```python
from build123d import *

# Parameters (mm, degrees)
SKETCH1_W                                       = 60
SKETCH1_H                                       = 120
BOSS_EXTRUDE1_DEPTH                             = 6.54
BOSS_EXTRUDE4_DEPTH                             = 27
SKETCH10_W                                      = 6.54
SKETCH10_H                                      = 45
BOSS_EXTRUDE5_DEPTH                             = 20
SKETCH17_W                                      = 60
SKETCH17_H                                      = 40
BOSS_EXTRUDE6_DEPTH                             = 29
CUT_EXTRUDE1_REACH                              = 72
SKETCH18_RX                                     = 20.2
SKETCH18_RY                                     = 12
CUT_EXTRUDE2_REACH                              = 57.54
SKETCH21_W                                      = 40.3853088
SKETCH21_H                                      = 40
SKETCH23_W                                      = 2
SKETCH23_H                                      = 36
CUT_EXTRUDE3_DEPTH                              = 9
SKETCH24_W                                      = 2
SKETCH24_H                                      = 36
CUT_EXTRUDE4_DEPTH                              = 9
CSK_FOR_M3_FLAT_HEAD_MACHINE_SCREW4_D           = 4.93
CSK_FOR_M3_FLAT_HEAD_MACHINE_SCREW4_DEPTH       = 6.54
CSK_FOR_M3_FLAT_HEAD_MACHINE_SCREW4_CSINK_D     = 12
CSK_FOR_M3_FLAT_HEAD_MACHINE_SCREW4_CSINK_ANGLE = 90
CSK_FOR_M3_FLAT_HEAD_MACHINE_SCREW5_D           = 4.93
CSK_FOR_M3_FLAT_HEAD_MACHINE_SCREW5_DEPTH       = 6.54
CSK_FOR_M3_FLAT_HEAD_MACHINE_SCREW5_CSINK_D     = 12
CSK_FOR_M3_FLAT_HEAD_MACHINE_SCREW5_CSINK_ANGLE = 90


with BuildPart() as part:
    # Sketch1 → Boss-Extrude1 (new body)
    with BuildSketch(Plane.XY):
        Rectangle(SKETCH1_W, SKETCH1_H)
    extrude(amount=BOSS_EXTRUDE1_DEPTH)

    # Sketch7 → Boss-Extrude4 (add)
    with BuildSketch(Plane.XY.offset(6.54)):
        with BuildLine():
            Line((-30, 44.483314774), (-30, 29.516685226))
            ThreePointArc((-30, 29.516685226), (-16, 37), (-30, 44.483314774))
        make_face()
    extrude(amount=BOSS_EXTRUDE4_DEPTH)

    # Sketch10 → Boss-Extrude5 (add)
    with BuildSketch(Plane(origin=(0, 0, 0), x_dir=(-1, 0, 0), z_dir=(0, 0, -1))):
        with Locations((23.27, -2.5)):
            Rectangle(SKETCH10_W, SKETCH10_H)
        with Locations((-23.27, -2.5)):
            Rectangle(SKETCH10_W, SKETCH10_H)
    extrude(amount=BOSS_EXTRUDE5_DEPTH)

    # Sketch17 → Boss-Extrude6 (add)
    with BuildSketch(Plane.XY.offset(6.54)):
        with Locations((0, -10)):
            Rectangle(SKETCH17_W, SKETCH17_H)
    extrude(amount=BOSS_EXTRUDE6_DEPTH)

    # Sketch18 → Cut-Extrude1 (cut, up to next)
    with BuildSketch(Plane(origin=(0, 10, 0), x_dir=(1, 0, 0), z_dir=(0, 1, 0)), mode=Mode.PRIVATE) as cut_extrude1_sk1:
        with Locations(Location((4.192654401, -20.096314851), (0, 0, 1.545214336))):
            Ellipse(SKETCH18_RX, SKETCH18_RY)
    cut_extrude1_tool1 = extrude(cut_extrude1_sk1.sketch, amount=-CUT_EXTRUDE1_REACH, mode=Mode.PRIVATE) & part.part
    add(cut_extrude1_tool1.solids().sort_by_distance((4.192654, 10, 20.096315))[0], mode=Mode.SUBTRACT)

    # Sketch21 → Cut-Extrude2 (cut, up to next)
    with BuildSketch(Plane.XY.offset(35.54), mode=Mode.PRIVATE) as cut_extrude2_sk1:
        with Locations((4.1926544, -10)):
            Rectangle(SKETCH21_W, SKETCH21_H)
    cut_extrude2_tool1 = extrude(cut_extrude2_sk1.sketch, amount=-CUT_EXTRUDE2_REACH, mode=Mode.PRIVATE) & part.part
    add(cut_extrude2_tool1.solids().sort_by_distance((4.192654, -10, 35.54))[0], mode=Mode.SUBTRACT)

    # Sketch23 → Cut-Extrude3 (cut)
    with BuildSketch(Plane(origin=(-16, 0, 0), x_dir=(0, 0, -1), z_dir=(1, 0, 0))):
        with Locations((-33.14, -10)):
            Rectangle(SKETCH23_W, SKETCH23_H)
    extrude(amount=-CUT_EXTRUDE3_DEPTH, mode=Mode.SUBTRACT)

    # Sketch24 → Cut-Extrude4 (cut)
    with BuildSketch(Plane.ZY.offset(-24.3853088)):
        with Locations((33.14, -10)):
            Rectangle(SKETCH24_W, SKETCH24_H)
    extrude(amount=-CUT_EXTRUDE4_DEPTH, mode=Mode.SUBTRACT)

    # CSK for M3 Flat Head Machine Screw4
    with Locations(Plane(origin=(26.54, -12.5, -10), x_dir=(0, 1, 0), z_dir=(1, 0, 0))):
        with Locations((0, 0), (20, 0)):
            CounterSinkHole(CSK_FOR_M3_FLAT_HEAD_MACHINE_SCREW4_D / 2, CSK_FOR_M3_FLAT_HEAD_MACHINE_SCREW4_CSINK_D / 2, depth=CSK_FOR_M3_FLAT_HEAD_MACHINE_SCREW4_DEPTH, counter_sink_angle=CSK_FOR_M3_FLAT_HEAD_MACHINE_SCREW4_CSINK_ANGLE)

    # CSK for M3 Flat Head Machine Screw5
    with Locations(Plane(origin=(-26.54, -12.5, -10), x_dir=(0, -1, 0), z_dir=(-1, 0, 0))):
        with Locations((0, 0), (-20, 0)):
            CounterSinkHole(CSK_FOR_M3_FLAT_HEAD_MACHINE_SCREW5_D / 2, CSK_FOR_M3_FLAT_HEAD_MACHINE_SCREW5_CSINK_D / 2, depth=CSK_FOR_M3_FLAT_HEAD_MACHINE_SCREW5_DEPTH, counter_sink_angle=CSK_FOR_M3_FLAT_HEAD_MACHINE_SCREW5_CSINK_ANGLE)


solid = part.part
```
For this review, take the finished solid that the model builds, in its own axes (mm). A direction names the side the tool comes from. Coordinates: 2 decimals unless noted, no trailing zeros. Write each loop counter-clockwise with the first axis right and the second up, starting at its lowest first coordinate (ties: lowest second). Pieces come first, ordered by that corner, then holes. Notation, with made-up numbers: (71, -17) - (78, -17) arc R32 ccw to (78, 14) - close; hole circle Ø5 at (-12.75, 28.5). An arc over 180 degrees is marked (long way). Answer in a Markdown table with one row per item. Add a question column.
Q1. We need section B-B, the plane y = 37. State the section outline as (x, z) points, and give its area (3 significant figures).
Q2. For probe 1 along Y at (x, z) = (-22.1, -10) (3 decimals); probe 2 along X at (y, z) = (2.5, -2); probe 3 along X at (y, z) = (-2.5, 33), list the stretches that pass through material, from the lowest coordinate up.
Q3. Draft analysis for pull direction Z (two halves, no side actions). For faces 1 (the conical face through (23.177, 8.072, -12.574)), 2 (the flat face through (27, -10, 35.54)), 3 (the cylindrical face through (-16, 37, 20)), state which applies: +Z half, -Z half, draft (parallel to the pull), parting line (faces both ways), or undercut.
Q4. Tool access review of faces 4 (the flat face through (24.385, -10, 28)), 5 (the flat face through (-20, -10, 34.14)), 6 (the flat face through (23, -25, -10)), 7 (the flat face through (20, -3, -10)): name each direction out of +Z, -Z, +X, -X, +Y, -Y from which nothing blocks a thin tool from reaching the whole face with its end or side.
Q5. We need section A-A, the plane z = -10. Count the separate pieces of the cut face and the enclosed holes in it, and give its area (3 significant figures).
Q6. For P1, Ø1, axis at x = 27.5, z = 33.5, coming from the +Y side; P2, Ø22, axis at y = -5.5, z = -12.5, coming from the +X side; P3, Ø2, axis at x = 4.5, y = 24, coming from the -Z side, all flat-tipped, find the tip position at first contact; note any pin that passes through.
Answer list:
| question | item | result |
|---|---|---|
| 1 | outline | (-30, 0) - (30, 0) - (30, 6.54) - (-16, 6.54) - (-16, 33.54) - (-30, 33.54) - close |
| 1 | area | 770 mm2 |
| 2 | probe 1 | y = -25 to -14.965, -10.035 to 5.035, 9.965 to 20 |
| 2 | probe 2 | x = -26.54 to -20, 20 to 26.54 |
| 2 | probe 3 | x = -30 to -25 |
| 3 | face 1 | undercut |
| 3 | face 2 | +Z half |
| 3 | face 3 | draft |
| 4 | face 4 | +Z, +Y, -Y |
| 4 | face 5 | +X |
| 4 | face 6 | -Z, +X, -X, -Y |
| 4 | face 7 | -Z, +Y, -Y |
| 5 | separate pieces | 6 |
| 5 | enclosed holes | 0 |
| 5 | area | 410 mm2 |
| 6 | P1 | stops at y = 10 |
| 6 | P2 | stops at x = 26.54 |
| 6 | P3 | stops at z = 0 |
